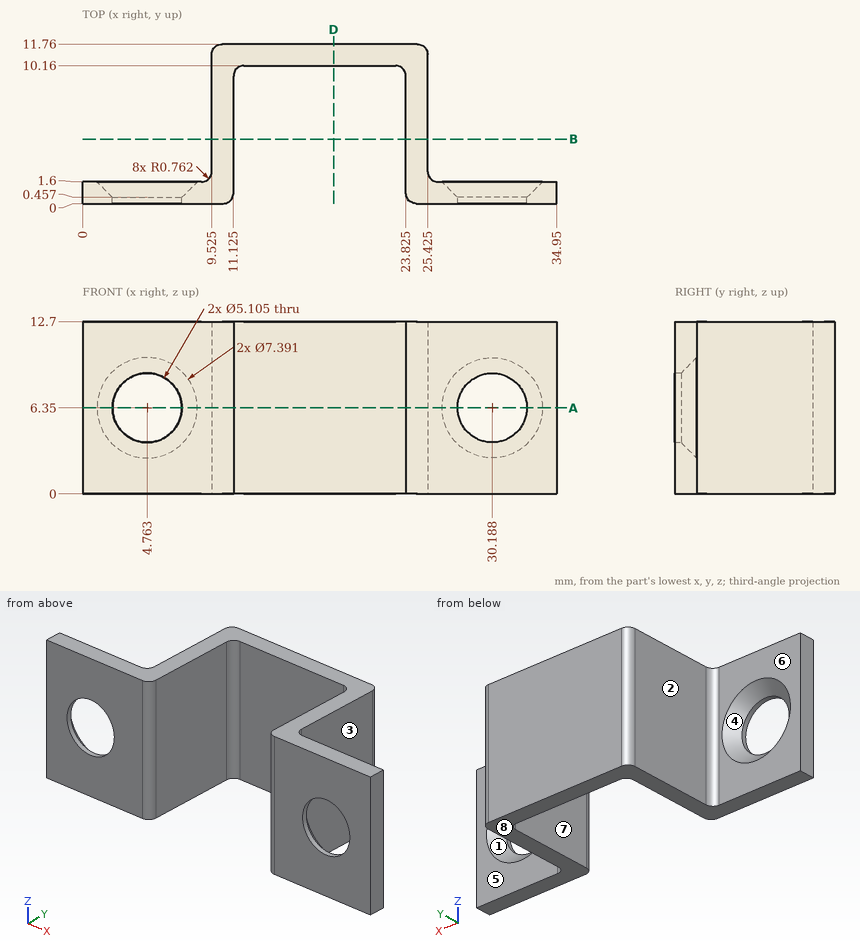
Verification items for this drawing (mm, ordinates from the low corner). A direction names the side the tool comes from. Round coordinates to 2 decimals unless told otherwise and drop trailing zeros. Write each loop counter-clockwise with the first axis right and the second up, starting at its lowest first coordinate (ties: lowest second). Pieces come first, ordered by that corner, then holes. Notation, with made-up numbers: M 82.25,44.5 L 113.25,44.5 A20 cw 113.25,71.5 Z; hole C -36,-7.5 d7. An arc over 180 degrees is marked long. Write item = value, one per line. Start each with the question number.
1. Gauge pin test, flat ends, axial feed: pin 1 (2.5 mm diameter, centred on y = 5.5, z = 7.5, fed in from -X) (1 decimal); pin 2 (2.5 mm diameter, centred on x = 30.5, z = 9.5, fed in from +Y); pin 3 (2.5 mm diameter, centred on y = 7.5, z = 5, fed in from +X) (1 decimal); pin 4 (6 mm diameter, centred on x = 26, y = 8.5, fed in from +Z). Record the tip position at first contact, or that the pin passes through.
2. Scan lines: line 1 (X direction, y = 3.5, z = 9.75) (1 decimal); line 2 (X direction, y = 10.75, z = 1.25) (1 decimal); line 3 (Y direction, x = 18.5, z = 2). Record each from-to range of solid material in increasing order. Write a range as [from, to].
3. Release check for a two-part mould opening along X. For the marked faces 1, 2 and 3 record: pulls with the +X half, pulls with the -X half, needs draft (parallel to the pull), parting line crosses it, or undercut.
4. Section check A-A, the plane z = 6.35. State how many separate pieces and enclosed holes the cut face has.
5. Section check D-D, the plane x = 18.5. Record the cut outline in (y, z).
6. Tool access check on the marked faces 4, 5, 6, 7 and 8. Record the directions out of +Z, -Z, +X, -X, +Y, -Y that give a thin tool (end or side, any length) a straight path to the whole face; none if there is none.
7. Section check B-B, the plane y = 4.75. Record the cut outline in (x, z) (1 decimal).
Results found:
q1.pin_1 = 9.5
q1.pin_2 = 1.6
q1.pin_3 = 25.4
q1.pin_4 = 12.7
q2.line_1 = [9.5, 11.1], [23.8, 25.4]
q2.line_2 = [9.5, 25.4]
q2.line_3 = [10.16, 11.76]
q3.face_1 = undercut
q3.face_2 = pulls with the -X half
q3.face_3 = pulls with the +X half
q4.separate_pieces = 3
q4.enclosed_holes = 0
q5.outline = M 10.16,0 L 11.76,0 L 11.76,12.7 L 10.16,12.7 Z
q6.face_4 = +Y
q6.face_5 = +Z, -Z, +X, +Y
q6.face_6 = +Z, -Z, -X, +Y
q6.face_7 = +Z, -Z, -Y
q6.face_8 = -Z, +X, -X, +Y, -Y
q7.outline = M 9.5,0 L 11.1,0 L 11.1,12.7 L 9.5,12.7 Z; M 23.8,0 L 25.4,0 L 25.4,12.7 L 23.8,12.7 Z
